Can you work these out from the model? Positions are in its coordinate system, mm. A direction names the side the tool comes from. Coordinates: 2 decimals unless noted, no trailing zeros. Loops run counter-clockwise (first coordinate to the right, second up) from the corner with the lowest first, then second, coordinate; pieces in that order, holes last. Notation, with made-up numbers: M 47,53.25 L 80,53.25 A19 ccw 80,80.25 Z; hole C 64,-19 d5. An arc over 180 degrees is marked long. Return JSON: item names as keys, results as strings. Group by question number.
```python
from build123d import *

# Parameters (mm, degrees)
SKETCH_1_R          = 2.15
SKETCH_1_R_2        = 6
SKETCH_1_R_3        = 3
SKETCH_1_R_4        = 1.6
EXTRUDE_1_DEPTH     = 3
CUT_EXTRUDE_1_DEPTH = 3
FILLET_1_R          = 2
FILLET_2_R          = 3


with BuildPart() as part:
    # ｽｹｯﾁ1 → ﾎﾞｽ - 押し出し1 (new body)
    with BuildSketch(Plane(origin=(0, 0, 0), x_dir=(0, 0, -1), z_dir=(1, 0, 0))):
        with BuildLine():
            Line((0, 0), (20, 0))
            Line((20, 0), (100.357645767, 34.814697588))
            ThreePointArc((100.357645767, 34.814697588), (101.226596702, 35.299021126), (101.982464697, 35.94578893))
            Line((101.982464697, 35.94578893), (125, 60))
            Line((125, 60), (125, 70))
            Line((125, 70), (106.736076333, 88.580227744))
            ThreePointArc((106.736076333, 88.580227744), (106.067997995, 89.149910996), (105.310570653, 89.593950967))
            Line((105.310570653, 89.593950967), (20, 130))
            Line((20, 130), (0, 130))
            Line((0, 130), (0, 0))
        make_face()
        with Locations((7.5, 120)):
            Circle(SKETCH_1_R, mode=Mode.SUBTRACT)
        with Locations((7.5, 90)):
            Circle(SKETCH_1_R, mode=Mode.SUBTRACT)
        with Locations(Location((7.5, 40, 0), (0, 0, 180))):
            Circle(SKETCH_1_R, mode=Mode.SUBTRACT)
        with Locations(Location((7.5, 10, 0), (0, 0, 180))):
            Circle(SKETCH_1_R, mode=Mode.SUBTRACT)
        with Locations((74.5, 65)):
            Circle(SKETCH_1_R_2, mode=Mode.SUBTRACT)
        with Locations((29.5, 65)):
            Circle(SKETCH_1_R_3, mode=Mode.SUBTRACT)
        with Locations((103.17032155, 85.075175272)):
            Circle(SKETCH_1_R, mode=Mode.SUBTRACT)
        with Locations((98.369942602, 39.402620443)):
            Circle(SKETCH_1_R, mode=Mode.SUBTRACT)
        with Locations((74.5, 81.215)):
            Circle(SKETCH_1_R_4, mode=Mode.SUBTRACT)
        with Locations(Location((74.5, 48.785, 0), (0, 0, 180))):
            Circle(SKETCH_1_R_4, mode=Mode.SUBTRACT)
        with Locations((105, 65)):
            Circle(SKETCH_1_R, mode=Mode.SUBTRACT)
        with Locations((120, 65)):
            Circle(SKETCH_1_R, mode=Mode.SUBTRACT)
    extrude(amount=EXTRUDE_1_DEPTH)

    # ｽｹｯﾁ2 → ｶｯﾄ - 押し出し1 (cut)
    with BuildSketch(Plane(origin=(3, 0, 0), x_dir=(0, 0, -1), z_dir=(1, 0, 0))):
        with BuildLine():
            Line((20, 113.402584003), (20, 72.399324293))
            ThreePointArc((20, 72.399324293), (25.68439104, 90.338435663), (37.083419962, 105.311283015))
            Line((37.083419962, 105.311283015), (20, 113.402584003))
        make_face()
        with BuildLine():
            Line((20, 16.347267022), (37.782097447, 24.051304879))
            ThreePointArc((37.782097447, 24.051304879), (25.904048448, 39.242797265), (20, 57.600675707))
            Line((20, 57.600675707), (20, 16.347267022))
        make_face()
    extrude(amount=-CUT_EXTRUDE_1_DEPTH, mode=Mode.SUBTRACT)

    # ﾌｨﾚｯﾄ1
    fillet_1_edges = [part.edges().sort_by_distance(p)[0] for p in [
        (1.5, 130, 0),
        (1.5, 130, -20),
        (1.5, 70, -125),
        (1.5, 60, -125),
        (1.5, 0, -20),
        (1.5, 0, 0),
    ]]
    fillet(fillet_1_edges, radius=FILLET_1_R)

    # ﾌｨﾚｯﾄ2
    fillet_2_edges = [part.edges().sort_by_distance(p)[0] for p in [
        (1.5, 105.311283015, -37.083419962),
        (1.5, 72.399324293, -20),
        (1.5, 113.402584003, -20),
        (1.5, 57.600675707, -20),
        (1.5, 24.051304879, -37.782097447),
        (1.5, 16.347267022, -20),
    ]]
    fillet(fillet_2_edges, radius=FILLET_2_R)


solid = part.part
```
1) If we mould it in two halves opening along Y, with no side actions, what happens to faces 3 (the face through (1.479, 65.264, -68.506)), 4 (the face through (1, 66, 0)), 5 (the face through (1, 0, -11))? For each: +Y half, -Y half, draft (parallel to the pull), parting line (faces both ways), or undercut.
2) For faces 1 (the face through (2, 30, -20)), 2 (the face through (3, 66, -48)), which set-ups out of +Z, -Z, +X, -X, +Y, -Y let a thin tool reach every point of the face, with its end or its side?
3) Suppose I cut it at B-B, the plane z = -7.5. List the corners of the cut face in (x, y) for me.
4) Suppose I cut it at A-A, the plane y = 65. List the corners of the cut face in (x, z) for me.
5) Suppose I cut it at C-C, the plane z = -74.5. List the corners of the cut face in (x, y) for me (3 decimals), then the cut area to 3 significant figures.
6) For pin 1 (11 mm diameter, centred on y = 65, z = -74.5, fed in from +X); pin 2 (1.5 mm diameter, centred on x = 2, z = -60, fed in from +Y), each with a flat end and sliding along its axis, tell me the tip position at first contact or that it passes through.
7) Suppose I cut it at D-D, the plane z = -120. List the corners of the cut face in (x, y) for me, then the cut area to 3 significant figures.
8) If I drill on line 1 (Y direction, x = 1.9, z = -7.5); line 2 (Y direction, x = 2.6, z = -74.5) (3 decimals); line 3 (Y direction, x = 0.65, z = -29.5), over which ranges is the centre line in solid material (lowest first)? Write a range as from..to.
Returned:
{
 "1": {"face 3": "undercut", "face 4": "draft", "face 5": "-Y half"},
 "2": {"face 1": "+X, -X", "face 2": "+Z, -Z, +X, +Y, -Y"},
 "3": {"outline": "M 0,0 L 3,0 L 3,7.85 L 0,7.85 Z; M 0,12.15 L 3,12.15 L 3,37.85 L 0,37.85 Z; M 0,42.15 L 3,42.15 L 3,87.85 L 0,87.85 Z; M 0,92.15 L 3,92.15 L 3,117.85 L 0,117.85 Z; M 0,122.15 L 3,122.15 L 3,130 L 0,130 Z"},
 "4": {"outline": "M 0,-125 L 3,-125 L 3,-122.15 L 0,-122.15 Z; M 0,-117.85 L 3,-117.85 L 3,-107.15 L 0,-107.15 Z; M 0,-102.85 L 3,-102.85 L 3,-80.5 L 0,-80.5 Z; M 0,-68.5 L 3,-68.5 L 3,-32.5 L 0,-32.5 Z; M 0,-26.5 L 3,-26.5 L 3,0 L 0,0 Z"},
 "5": {"outline": "M 0,23.612 L 3,23.612 L 3,47.185 L 0,47.185 Z; M 0,50.385 L 3,50.385 L 3,59 L 0,59 Z; M 0,71 L 3,71 L 3,79.615 L 0,79.615 Z; M 0,82.815 L 3,82.815 L 3,104.187 L 0,104.187 Z", "area": "187 mm²"},
 "6": {"pin 1": "passes through", "pin 2": "stops at y = 111.41"},
 "7": {"outline": "M 0,54.77 L 3,54.77 L 3,62.85 L 0,62.85 Z; M 0,67.15 L 3,67.15 L 3,75.09 L 0,75.09 Z", "area": "48.0 mm²"},
 "8": {"line 1": "y = 0..7.85, 12.15..37.85, 42.15..87.85, 92.15..117.85, 122.15..130", "line 2": "y = 23.612..47.185, 50.385..59, 71..79.615, 82.815..104.187", "line 3": "y = 4.12..20.46, 33.38..62, 68..96.62, 108.9..125.5"}
}
